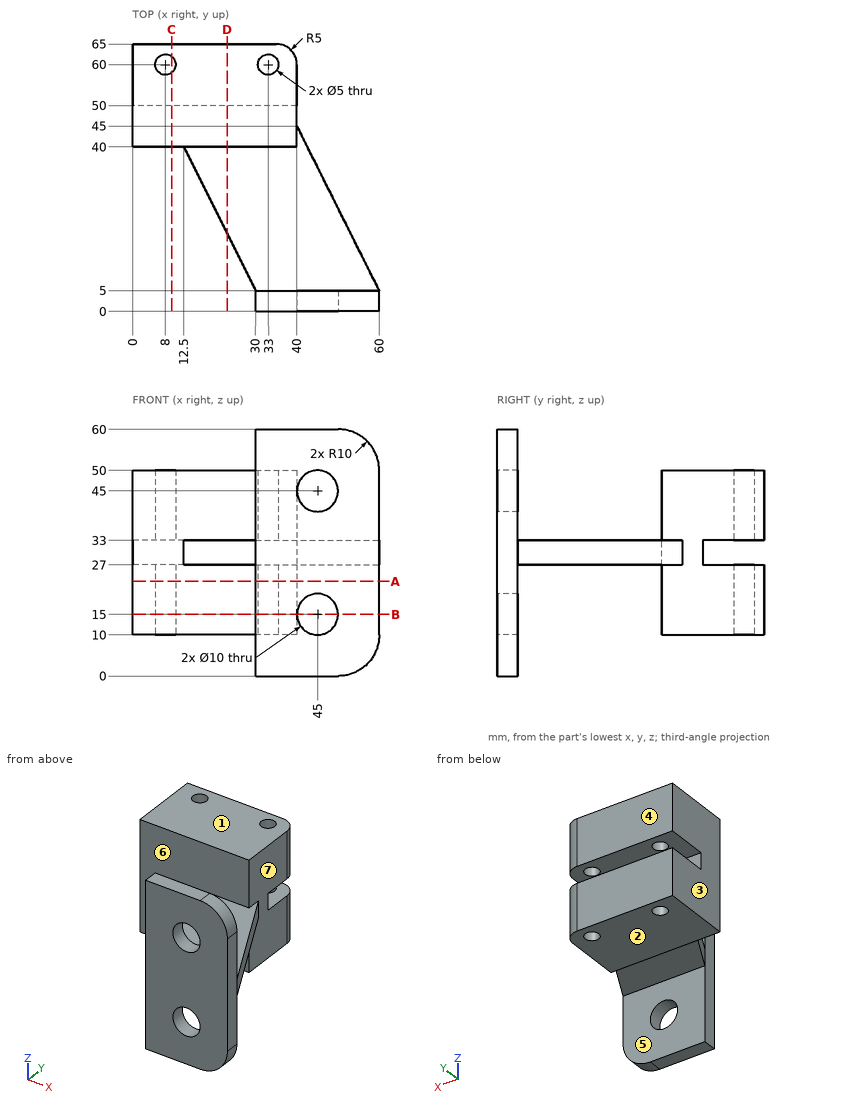
Geometry: see drawing. Coordinates: mm, zero at the bounding-box minimum. A direction names the side the tool comes from. Coordinates: 2 decimals unless noted, no trailing zeros. Order: outer loops, then holes, each group sorted by start corner. A loop starts at its lowest first (then second) coordinate and runs counter-clockwise, first axis right, second up. Notation, with made-up numbers: (78, 1.25) - (127, 1.25) arc R21 ccw to (127, 15.25) - close; hole circle Ø11 at (75.5, -10.5). An arc over 180 degrees is marked (long way). Use one line per item in the form item = value.
1) Mould query, pull axis Y, two halves, no side actions, for the marked faces 4, 5, 6 and 7. Classes: +Y half, -Y half, draft (parallel to the pull), parting line (faces both ways), or undercut.
Solutions:
face_4 = +Y half
face_5 = undercut
face_6 = undercut
face_7 = draft
2) Section B-B (z = 15). Return loops of the section in (x, y), then the cut area to 3 significant figures.
Solutions:
outline = (0, 40) - (40, 40) - (40, 60) arc R5 ccw to (35, 65) - (0, 65) - close; (30, 0) - (40, 0) - (40, 5) - (30, 5) - close; (50, 0) - (60, 0) - (60, 5) - (50, 5) - close; hole circle Ø5 at (8, 60); hole circle Ø5 at (33, 60)
area = 1,060 mm^2
3) Section A-A (z = 23). Return loops of the section in (x, y), then the cut area to 3 significant figures.
Solutions:
outline = (0, 40) - (40, 40) - (40, 60) arc R5 ccw to (35, 65) - (0, 65) - close; (30, 0) - (60, 0) - (60, 5) - (30, 5) - close; hole circle Ø5 at (8, 60); hole circle Ø5 at (33, 60)
area = 1,110 mm^2
4) Ray query, L1, parallel to Y at x = 33, z = 45; L2, parallel to X at y = 2, z = 15; L3, parallel to Y at x = 8, z = 17. Return the intervals inside material, ascending.
Solutions:
L1 = 0 to 5, 40 to 57.5, 62.5 to 65
L2 = 30 to 40, 50 to 60
L3 = 40 to 57.5, 62.5 to 65
5) Set-up query: the marked faces 1, 2 and 3. Return all of +Z, -Z, +X, -X, +Y, -Y with unobstructed straight access to the full face (end or side cutting, diameter ignored); none if empty.
Solutions:
face_1 = +Z, +X, -X, +Y
face_2 = -Z, +X, -X, +Y
face_3 = +Z, -Z, -X, +Y, -Y
6) Section D-D (x = 23). Return loops of the section in (y, z), then the cut area to 3 significant figures.
Solutions:
outline = (19, 27) - (40, 27) - (40, 10) - (65, 10) - (65, 27) - (50, 27) - (50, 33) - (65, 33) - (65, 50) - (40, 50) - (40, 33) - (19, 33) - close
area = 1,040 mm^2
7) Section C-C (x = 9.5). Return loops of the section in (y, z), then the cut area to 3 significant figures.
Solutions:
outline = (40, 10) - (58, 10) - (58, 27) - (50, 27) - (50, 33) - (58, 33) - (58, 50) - (40, 50) - close; (62, 10) - (65, 10) - (65, 27) - (62, 27) - close; (62, 33) - (65, 33) - (65, 50) - (62, 50) - close
area = 774 mm^2
8) Pin query (flat end, axial travel): pin 1 (1.5 mm diameter, centred on x = 37, y = 54, fed in from +Z); pin 2 (6 mm diameter, centred on x = 42.5, y = 16.5, fed in from -Z); pin 3 (1.5 mm diameter, centred on y = 1.5, z = 42.5, fed in from -X). Return the tip coordinate at first contact, or that it passes through.
Solutions:
pin_1 = 50
pin_2 = 27
pin_3 = 30
